Check sheet for the modelled part. Datum: model origin and axes. Units: mm. Face numbers are marked on the shaded views. A direction names the side the tool comes from. Round coordinates to 2 decimals unless told otherwise and drop trailing zeros. Loops run counter-clockwise (first coordinate to the right, second up) from the corner with the lowest first, then second, coordinate; pieces in that order, holes last. Notation, with made-up numbers: (-26.5, 76) - (25.5, 76) arc R36 ccw to (25.5, 112) - close; hole circle Ø9 at (-38, -12). An arc over 180 degrees is marked (long way). Put each result on its own line as item: value.
```python
from build123d import *

# Parameters (mm, degrees)
ESQUISSE1_R             = 16
BOSS_EXTRU_1_DEPTH      = 1
ESQUISSE2_R             = 13
BOSS_EXTRU_2_DEPTH      = 8
ESQUISSE3_R             = 16
BOSS_EXTRU_3_DEPTH      = 1
ESQUISSE4_R             = 7
BOSS_EXTRU_4_DEPTH      = 5
ESQUISSE6_R             = 13
BOSS_EXTRU_5_DEPTH      = 0.5
ESQUISSE7_R             = 13
BOSS_EXTRU_6_DEPTH      = 0.5
ESQUISSE8_R             = 4
ENL_V_MAT_EXTRU_2_DEPTH = 16


with BuildPart() as part:
    # Esquisse1 → Boss.-Extru.1 (new body)
    with BuildSketch(Plane.XY):
        Circle(ESQUISSE1_R)
    extrude(amount=BOSS_EXTRU_1_DEPTH)

    # Esquisse2 → Boss.-Extru.2 (add)
    with BuildSketch(Plane.XY.offset(1)):
        Circle(ESQUISSE2_R)
    extrude(amount=BOSS_EXTRU_2_DEPTH)

    # Esquisse3 → Boss.-Extru.3 (add)
    with BuildSketch(Plane.XY.offset(9)):
        Circle(ESQUISSE3_R)
    extrude(amount=BOSS_EXTRU_3_DEPTH)

    # Esquisse4 → Boss.-Extru.4 (add)
    with BuildSketch(Plane.XY.offset(10)):
        Circle(ESQUISSE4_R)
    extrude(amount=BOSS_EXTRU_4_DEPTH)

    # Esquisse6 → Boss.-Extru.5 (add)
    with BuildSketch(Plane.XY.offset(10)):
        Circle(ESQUISSE6_R)
    extrude(amount=BOSS_EXTRU_5_DEPTH)

    # Esquisse7 → Boss.-Extru.6 (add)
    with BuildSketch(Plane(origin=(0, 0, 0), x_dir=(-1, 0, 0), z_dir=(0, 0, -1))):
        Circle(ESQUISSE7_R)
    extrude(amount=BOSS_EXTRU_6_DEPTH)

    # Esquisse8 → Enlèv. mat.-Extru.2 (cut)
    with BuildSketch(Plane.XY.offset(15)):
        Circle(ESQUISSE8_R)
    extrude(amount=-ENL_V_MAT_EXTRU_2_DEPTH, mode=Mode.SUBTRACT)


solid = part.part
```
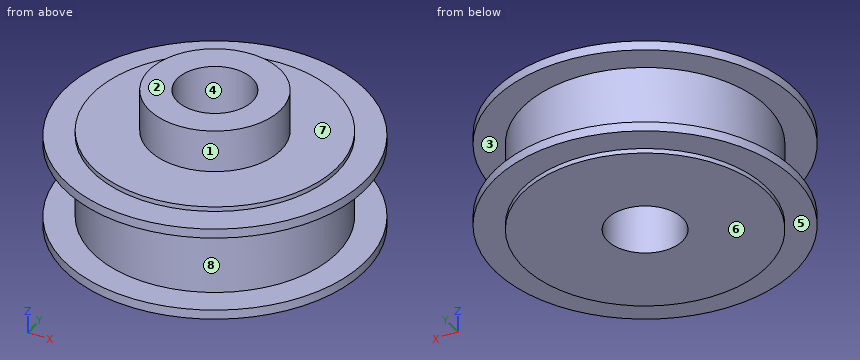
Item 1: Section check C-C on x = -2. Enter the section's corners in (y, z).
Filled sheet:
outline: (-15.87, 0) - (-12.85, 0) - (-12.85, -0.5) - (-3.46, -0.5) - (-3.46, 15) - (-6.71, 15) - (-6.71, 10.5) - (-12.85, 10.5) - (-12.85, 10) - (-15.87, 10) - (-15.87, 9) - (-12.85, 9) - (-12.85, 1) - (-15.87, 1) - close; (3.46, -0.5) - (12.85, -0.5) - (12.85, 0) - (15.87, 0) - (15.87, 1) - (12.85, 1) - (12.85, 9) - (15.87, 9) - (15.87, 10) - (12.85, 10) - (12.85, 10.5) - (6.71, 10.5) - (6.71, 15) - (3.46, 15) - close
Item 2: Thickness scan on line 1 (Y direction, x = 0, z = 3.25); line 2 (Z direction, x = 0.5, y = 15); line 3 (Y direction, x = 0, z = 11). Record the ranges inside material, lowest first. Write a range as from..to.
Filled sheet:
line 1: -13..-4, 4..13
line 2: 0..1, 9..10
line 3: -7..-4, 4..7
Item 3: Release check for a two-part mould opening along Z. For the marked faces 1, 2 and 3 record: +Z half, -Z half, draft (parallel to the pull), parting line (faces both ways), or undercut.
Filled sheet:
face 1: draft
face 2: +Z half
face 3: undercut
Item 4: Section check D-D on y = -10. Enter the section's corners in (x, z).
Filled sheet:
outline: (-12.49, 0) - (-8.31, 0) - (-8.31, -0.5) - (8.31, -0.5) - (8.31, 0) - (12.49, 0) - (12.49, 1) - (8.31, 1) - (8.31, 9) - (12.49, 9) - (12.49, 10) - (8.31, 10) - (8.31, 10.5) - (-8.31, 10.5) - (-8.31, 10) - (-12.49, 10) - (-12.49, 9) - (-8.31, 9) - (-8.31, 1) - (-12.49, 1) - close
Item 5: Section check A-A on y = 0. Enter the section's corners in (x, z).
Filled sheet:
outline: (-16, 0) - (-13, 0) - (-13, -0.5) - (-4, -0.5) - (-4, 15) - (-7, 15) - (-7, 10.5) - (-13, 10.5) - (-13, 10) - (-16, 10) - (-16, 9) - (-13, 9) - (-13, 1) - (-16, 1) - close; (4, -0.5) - (13, -0.5) - (13, 0) - (16, 0) - (16, 1) - (13, 1) - (13, 9) - (16, 9) - (16, 10) - (13, 10) - (13, 10.5) - (7, 10.5) - (7, 15) - (4, 15) - close
Item 6: Section check B-B on z = 11. Enter the section's corners in (x, y).
Filled sheet:
outline: circle Ø14 at (0, 0); hole circle Ø8 at (0, 0)
Item 7: Tool access check on the marked faces 4, 5, 6, 7 and 8. Record the directions out of +Z, -Z, +X, -X, +Y, -Y that give a thin tool (end or side, any length) a straight path to the whole face; none if there is none.
Filled sheet:
face 4: +Z, -Z
face 5: -Z
face 6: -Z, +X, -X, +Y, -Y
face 7: +Z
face 8: none
Item 8: Go/stop test with flat-tipped pins: pin 1 (8 mm diameter, centred on x = 3, z = 13, fed in from -Y); pin 2 (8 mm diameter, centred on y = 10, z = 8.5, fed in from -X); pin 3 (1 mm diameter, centred on y = 6, z = 7.5, fed in from -X). Record where each tip stops, or that it passes through.
Filled sheet:
pin 1: y = -16
pin 2: x = -14.82
pin 3: x = -11.78
